Here's the drawing with two shaded views (mm, measured from the low corner). I have some questions. A direction names the side the tool comes from. Coordinates: 2 decimals unless noted, no trailing zeros. Order: outer loops, then holes, each group sorted by start corner. A loop starts at its lowest first (then second) coordinate and runs counter-clockwise, first axis right, second up. Notation, with made-up numbers: M 59,1 L 91,1 A22 ccw 91,25 Z; hole C 41,40.5 d8. An arc over 180 degrees is marked long. Put each result on its own line as item: value. Start each with the question number.
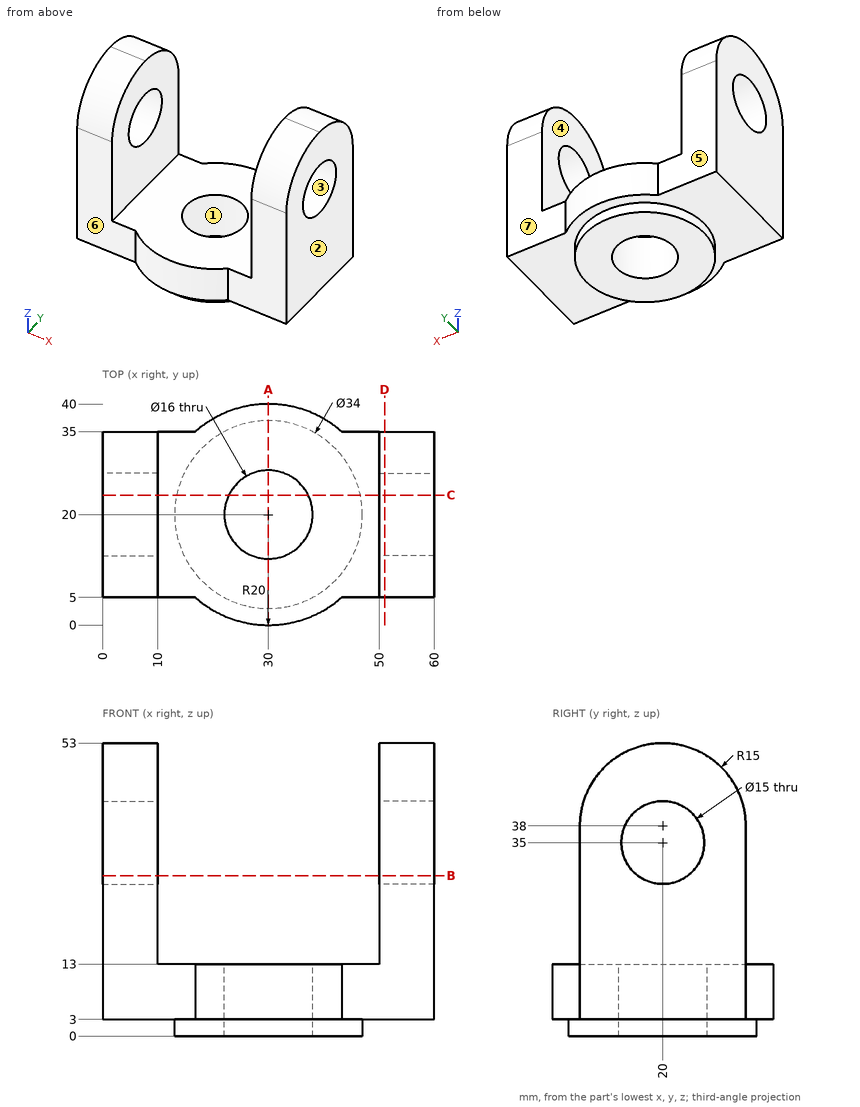
Item 1: I need wall thicknesses on probe 1 along Z at (x, y) = (2, 20); probe 2 along X at (y, z) = (9, 42.5); probe 3 along Y at (x, z) = (57, 35). Which ranges of each line are inside material? Lowest first, please.
Item 2: If we section it at B-B on z = 29: Write out the boundary of the cut face in (x, y).
Item 3: For the marked faces 5, 6 and 7, which set-ups out of +Z, -Z, +X, -X, +Y, -Y let a thin tool reach every point of the face, with its end or its side?
Item 4: If we section it at A-A on x = 30: Write out the boundary of the cut face in (y, z), then the cut area to 3 significant figures.
Item 5: If we mould it in two halves opening along X, with no side actions, what happens to the marked faces 1, 2, 3 and 4? For each: released by +X, released by -X, zero draft, split by the parting line, or undercut.
Item 6: If we section it at C-C on y = 23.5: Write out the boundary of the cut face in (x, z).
Item 7: If we section it at D-D on x = 51: Write out the boundary of the cut face in (y, z), then the cut area to 3 significant figures.
Item 8: For pin 1 Ø18.5 at (x, z) = (50, 16.5) entering from +Y; pin 2 Ø13.5 at (x, z) = (5, 12) entering from -Y; pin 3 Ø12 at (y, z) = (20, 35) entering from -X; pin 4 Ø5 at (x, z) = (10.5, 18) entering from +Y, each with a flat end and sliding along its axis, tell me the tip position at first contact or that it passes through.
Geometry check:
1. probe 1: z = 3 to 27.5, 42.5 to 53
1. probe 2: x = 0 to 10, 50 to 60
1. probe 3: y = 5 to 12.5, 27.5 to 35
2. outline: M 0,5 L 10,5 L 10,15.5 L 0,15.5 Z; M 0,24.5 L 10,24.5 L 10,35 L 0,35 Z; M 50,5 L 60,5 L 60,15.5 L 50,15.5 Z; M 50,24.5 L 60,24.5 L 60,35 L 50,35 Z
3. face 5: +Z, -Z, -X, +Y
3. face 6: +Z, -Z, -X, -Y
3. face 7: +Z, -Z, +X, +Y
4. outline: M 0,3 L 3,3 L 3,0 L 12,0 L 12,13 L 0,13 Z; M 28,0 L 37,0 L 37,3 L 40,3 L 40,13 L 28,13 Z
4. area: 294 mm²
5. face 1: undercut
5. face 2: released by +X
5. face 3: zero draft
5. face 4: undercut
6. outline: M 0,3 L 13.36,3 L 13.36,0 L 22.81,0 L 22.81,13 L 10,13 L 10,28.37 L 0,28.37 Z; M 0,41.63 L 10,41.63 L 10,52.59 L 0,52.59 Z; M 37.19,0 L 46.64,0 L 46.64,3 L 60,3 L 60,28.37 L 50,28.37 L 50,13 L 37.19,13 Z; M 50,41.63 L 60,41.63 L 60,52.59 L 50,52.59 Z
7. outline: M 5,3 L 35,3 L 35,38 A15 ccw 20,53 A15 ccw 5,38 Z; hole C 20,35 d15
7. area: 1,230 mm²
8. pin 1: stops at y = 36.41
8. pin 2: stops at y = 5
8. pin 3: passes through
8. pin 4: stops at y = 35
